Verification items for this drawing (mm, ordinates from the low corner). Give positions to 0.01 mm unless a question says otherwise; leave off trailing zeros. Order: outer loops, then holes, each group sorted by start corner. A loop starts at its lowest first (then second) coordinate and runs counter-clockwise, first axis right, second up.
(1) Sectioned sample at A-A on y = 30.48. Record the cut outline in (x, z) (1 decimal).
(2) Gauge pin test, flat ends, axial feed: pin 1 (2 mm diameter, centred on x = 19.5, z = 7.5, fed in from -Y); pin 2 (2 mm diameter, centred on y = 33.5, z = 7.5, fed in from +X); pin 3 (1 mm diameter, centred on y = 8.5, z = 5, fed in from -X) (1 decimal). Record the tip position at first contact, or that the pin passes through.
(3) Sectioned sample at B-B on x = 30.48. Record the cut outline in (y, z) (1 decimal).
(4) Scan lines: L1, parallel to Y at x = 30.48, z = 7 (1 decimal); L2, parallel to X at y = 34, z = 1.5 (1 decimal); L3, parallel to Y at x = 38, z = 9.75 (1 decimal). Record each from-to range of solid material in increasing order.
(5) Sectioned sample at D-D on y = 16. Record the cut outline in (x, z).
(6) Mould release check, pull along X, two halves, no side actions. Record for the marked faces 1, 2 and 3: pulls with the +X half, pulls with the -X half, needs draft (parallel to the pull), parting line crosses it, or undercut.
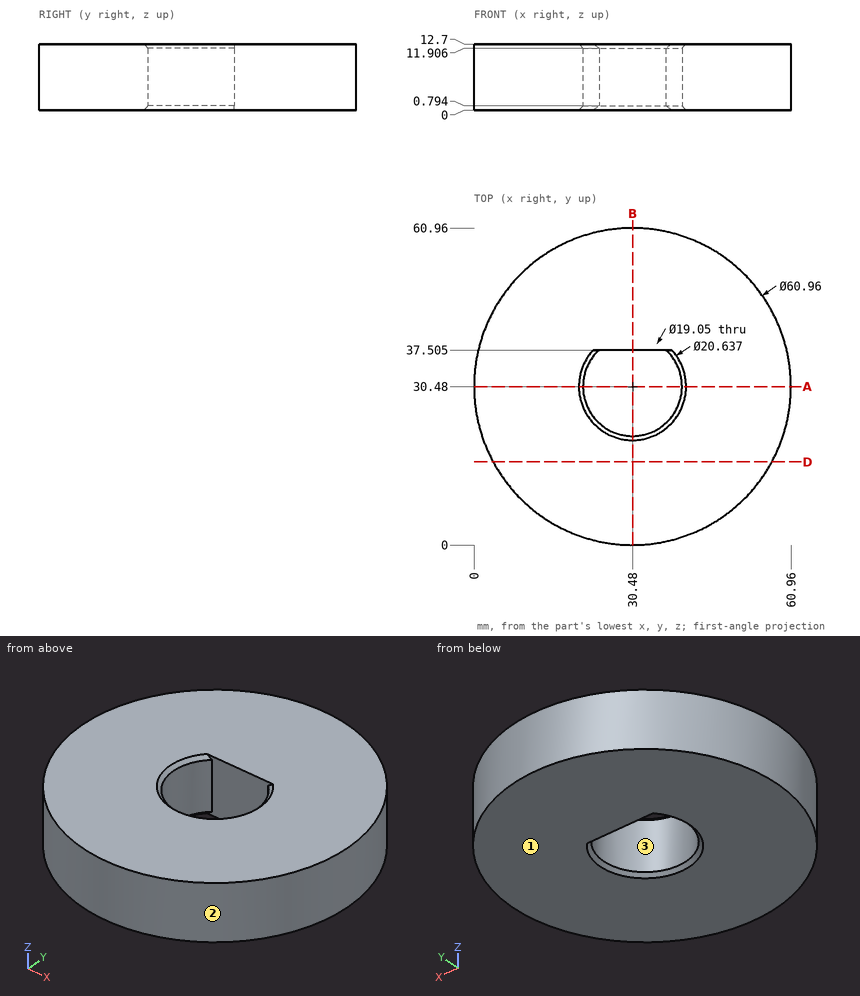
Ans:
1. outline: (0, 0) - (20.2, 0) - (21, 0.8) - (21, 11.9) - (20.2, 12.7) - (0, 12.7) - close; (40, 0.8) - (40.8, 0) - (61, 0) - (61, 12.7) - (40.8, 12.7) - (40, 11.9) - close
2. pin 1: stops at y = 1.68
2. pin 2: stops at x = 60.89
2. pin 3: stops at x = 8.9
3. outline: (0, 0) - (20.2, 0) - (21, 0.8) - (21, 11.9) - (20.2, 12.7) - (0, 12.7) - close; (37.5, 0) - (61, 0) - (61, 12.7) - (37.5, 12.7) - close
4. L1: y = 0 to 21, 37.5 to 61
4. L2: x = 0.2 to 21.6, 39.3 to 60.8
4. L3: y = 0.9 to 24.6, 36.3 to 60
5. outline: (3.66, 0) - (57.3, 0) - (57.3, 12.7) - (3.66, 12.7) - close
6. face 1: needs draft
6. face 2: parting line crosses it
6. face 3: undercut
